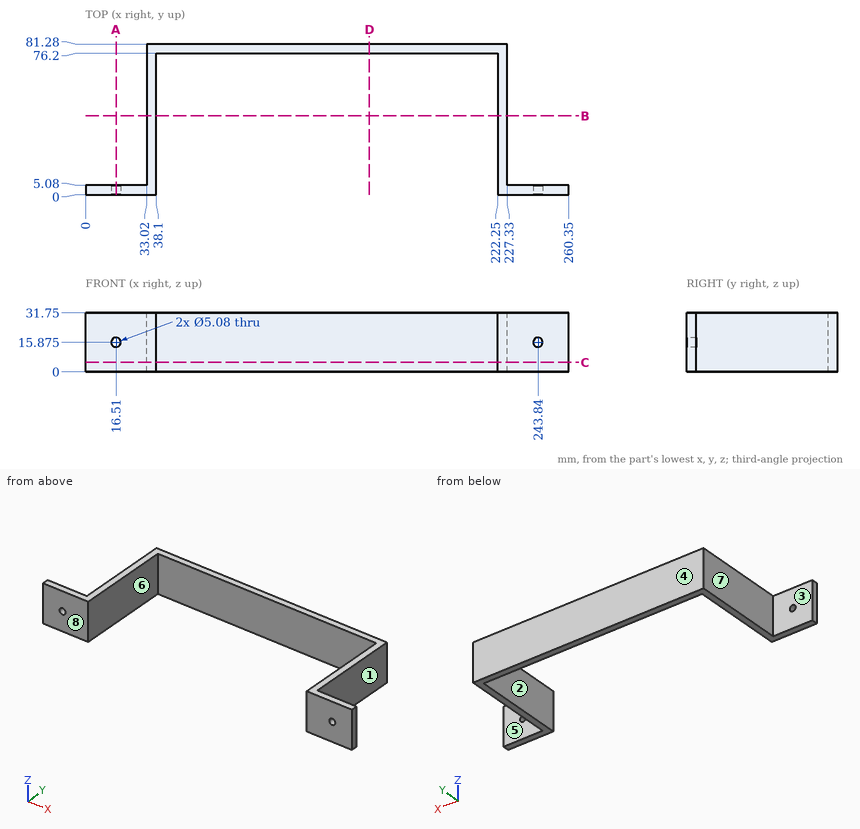
The drawing under review shows one solid part. Ordinate dimensions are in mm from its lowest x, y, z. A direction names the side the tool comes from. Give positions to 0.01 mm unless a question says otherwise; leave off trailing zeros. Write each loop counter-clockwise with the first axis right and the second up, starting at its lowest first coordinate (ties: lowest second). Pieces come first, ordered by that corner, then holes.
1. Add section D-D, the plane x = 153. Write out the cut boundary in (y, z), plus the area to 3 significant figures.
2. Wall thickness on L1, parallel to Z at x = 243.84, y = 2.05 (3 decimals); L2, parallel to X at y = 6, z = 24.5; L3, parallel to Z at x = 16, y = 1: over which ranges is each line inside the solid? List them lowest first.
3. Add section C-C, the plane z = 5. Write out the cut boundary in (x, y), plus the area to 3 significant figures.
4. For P1, Ø1, axis at y = 71.5, z = 18, coming from the -X side; P2, Ø10, axis at y = 63, z = 6.5, coming from the +X side; P3, Ø16, axis at x = 250, z = 19, coming from the +Y side; P4, Ø4, axis at x = 16.51, z = 15.875, coming from the -Y side (3 decimals), all flat-tipped, find the tip position at first contact; note any pin that passes through.
5. Tool access review of the marked faces 4, 5, 6, 7 and 8: name each direction out of +Z, -Z, +X, -X, +Y, -Y from which nothing blocks a thin tool from reaching the whole face with its end or side.
6. Add section A-A, the plane x = 16.51. Write out the cut boundary in (y, z) (3 decimals), plus the area to 3 significant figures.
7. Draft analysis for pull direction X (two halves, no side actions). For the marked faces 1, 2 and 3, state which applies: +X half, -X half, draft (parallel to the pull), parting line (faces both ways), or undercut.
8. Add section B-B, the plane y = 42.5. Write out the cut boundary in (x, z).
Worked answers:
1. outline: (76.2, 0) - (81.28, 0) - (81.28, 31.75) - (76.2, 31.75) - close
1. area: 161 mm2
2. L1: z = 0 to 13.335, 18.415 to 31.75
2. L2: x = 33.02 to 38.1, 222.25 to 227.33
2. L3: z = 0 to 13.39, 18.36 to 31.75
3. outline: (0, 0) - (38.1, 0) - (38.1, 76.2) - (222.25, 76.2) - (222.25, 0) - (260.35, 0) - (260.35, 5.08) - (227.33, 5.08) - (227.33, 81.28) - (33.02, 81.28) - (33.02, 5.08) - (0, 5.08) - close
3. area: 2,100 mm2
4. P1: stops at x = 33.02
4. P2: stops at x = 227.33
4. P3: stops at y = 5.08
4. P4: passes through
5. face 4: +Z, -Z, +X, -X, +Y
5. face 5: +Z, -Z, +X, +Y
5. face 6: +Z, -Z, -Y
5. face 7: +Z, -Z, -X, +Y
5. face 8: +Z, -Z, +X, -X, -Y
6. outline: (0, 0) - (5.08, 0) - (5.08, 13.335) - (0, 13.335) - close; (0, 18.415) - (5.08, 18.415) - (5.08, 31.75) - (0, 31.75) - close
6. area: 135 mm2
7. face 1: +X half
7. face 2: undercut
7. face 3: draft
8. outline: (33.02, 0) - (38.1, 0) - (38.1, 31.75) - (33.02, 31.75) - close; (222.25, 0) - (227.33, 0) - (227.33, 31.75) - (222.25, 31.75) - close
